from build123d import *

# Parameters (mm, degrees)
SKETCH_1_W          = 70
SKETCH_1_H          = 40
EXTRUDE_1_DEPTH     = 1.5
FILLET_1_R          = 3
SKETCH_2_W          = 13.5
SKETCH_2_H          = 20.4
CUT_EXTRUDE_1_DEPTH = 41.339186903
SKETCH_3_R          = 1
CUT_EXTRUDE_2_DEPTH = 41.339186903


with BuildPart() as part:
    # Эскиз1 → Бобышка-Вытянуть1 (new body)
    with BuildSketch(Plane(origin=(0, 0, 0), x_dir=(1, 0, 0), z_dir=(0, 1, 0))):
        Rectangle(SKETCH_1_W, SKETCH_1_H)
    extrude(amount=EXTRUDE_1_DEPTH)

    # Скругление1
    fillet_1_edges = [part.edges().sort_by_distance(p)[0] for p in [
        (-35, 0.75, -20),
        (35, 0.75, -20),
        (35, 0.75, 20),
        (-35, 0.75, 20),
    ]]
    fillet(fillet_1_edges, radius=FILLET_1_R)

    # Эскиз2 → Вырез-Вытянуть1 (cut, through all)
    with BuildSketch(Plane(origin=(0, 1.5, 0), x_dir=(1, 0, 0), z_dir=(0, 1, 0))):
        with Locations((28.25, 0)):
            Rectangle(SKETCH_2_W, SKETCH_2_H)
    extrude(amount=-CUT_EXTRUDE_1_DEPTH, mode=Mode.SUBTRACT)

    # Эскиз3 → Вырез-Вытянуть2 (cut, through all)
    with BuildSketch(Plane.XZ):
        with Locations(Location((19, -5, 0), (0, 0, 270))):
            Circle(SKETCH_3_R)
        with Locations(Location((19, 5, 0), (0, 0, 90))):
            Circle(SKETCH_3_R)
        with Locations(Location((32.5, -12.5, 0), (0, 0, 270))):
            Circle(SKETCH_3_R)
        with Locations(Location((32.5, 12.5, 0), (0, 0, 90))):
            Circle(SKETCH_3_R)
    extrude(amount=-CUT_EXTRUDE_2_DEPTH, mode=Mode.SUBTRACT)


solid = part.part
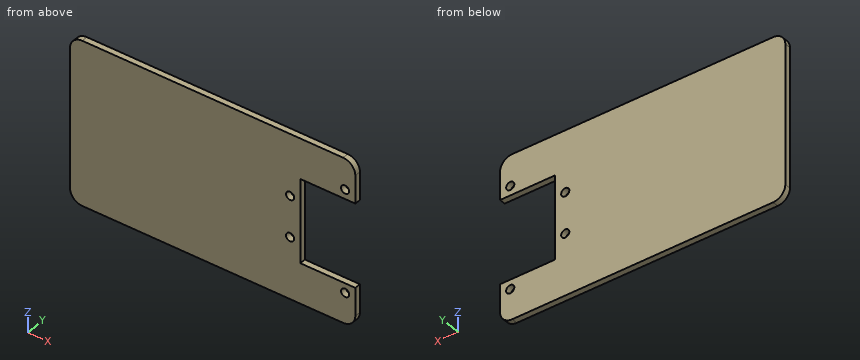
Here's how the part is built. I have some questions about the finished solid (model axes, mm). Round coordinates to 2 decimals unless told otherwise and drop trailing zeros. Order: outer loops, then holes, each group sorted by start corner. A loop starts at its lowest first (then second) coordinate and runs counter-clockwise, first axis right, second up. Notation, with made-up numbers: (77.25, 54.5) -> (104.25, 54.5) arc R24 cw to (104.25, 77.5) -> close; hole circle Ø8 at (38.25, 11.5). An arc over 180 degrees is marked (long way). Return JSON: item names as keys, results as strings.
Q1. If we section it at A-A on x = 27.5: List the corners of the cut face in (y, z) for me, plus the area to 3 significant figures.
Filled sheet:
{"outline": "(0, -20) -> (1.5, -20) -> (1.5, -10.2) -> (0, -10.2) -> close; (0, 10.2) -> (1.5, 10.2) -> (1.5, 20) -> (0, 20) -> close", "area": "29.4 mm^2"}
Q2. If we section it at B-B on y = 0.85: List the corners of the cut face in (x, z) for me.
Filled sheet:
{"outline": "(-35, -17) arc R3 ccw to (-32, -20) -> (32, -20) arc R3 ccw to (35, -17) -> (35, -10.2) -> (21.5, -10.2) -> (21.5, 10.2) -> (35, 10.2) -> (35, 17) arc R3 ccw to (32, 20) -> (-32, 20) arc R3 ccw to (-35, 17) -> close; hole circle Ø2 at (19, -5); hole circle Ø2 at (19, 5); hole circle Ø2 at (32.5, -12.5); hole circle Ø2 at (32.5, 12.5)"}
Q3. If we section it at C-C on z = -12.5: List the corners of the cut face in (x, y) for me, plus the area to 3 significant figures.
Filled sheet:
{"outline": "(-35, 0) -> (31.5, 0) -> (31.5, 1.5) -> (-35, 1.5) -> close; (33.5, 0) -> (35, 0) -> (35, 1.5) -> (33.5, 1.5) -> close", "area": "102 mm^2"}
Q4. I need wall thicknesses on line 1 along X through (y, z) = (0.95, 5); line 2 along Z through (x, y) = (26.5, 0.6); line 3 along X through (y, z) = (0.5, 12.5). Which ranges of each line are inside material? Lowest first, please. Write a range as from..to.
Filled sheet:
{"line 1": "x = -35..18, 20..21.5", "line 2": "z = -20..-10.2, 10.2..20", "line 3": "x = -35..31.5, 33.5..35"}
Q5. If we section it at D-D on x = 19: List the corners of the cut face in (y, z) for me.
Filled sheet:
{"outline": "(0, -20) -> (1.5, -20) -> (1.5, -6) -> (0, -6) -> close; (0, -4) -> (1.5, -4) -> (1.5, 4) -> (0, 4) -> close; (0, 6) -> (1.5, 6) -> (1.5, 20) -> (0, 20) -> close"}
